```python
from build123d import *

# Parameters (mm, degrees)
F0_W          = 1463
F0_H          = 50
F1_DEPTH      = 15
F1_DEPTH_BACK = 15
F3_DEPTH      = 50
F5_DEPTH      = 50


with BuildPart() as f1:
    # F0 (on Right) → F1 (new body, two sides)
    with BuildSketch(Plane.YZ) as f1_sk:
        Rectangle(F0_W, F0_H)
    extrude(amount=F1_DEPTH)
    extrude(f1_sk.sketch, amount=-F1_DEPTH_BACK)

    # F2 (on face) → F3 (join)
    with BuildSketch(Plane(origin=(0, 0, -25), x_dir=(1, 0, 0), z_dir=(0, 0, -1))):
        with BuildLine():
            ThreePointArc((0, 729.5), (-4.949747, 717.550253), (7, 722.5))
            ThreePointArc((7, 722.5), (4.949747, 727.449747), (0, 729.5))
        make_face()
    extrude(amount=F3_DEPTH)

    # F4 (on face) → F5 (join)
    with BuildSketch(Plane(origin=(0, 0, -25), x_dir=(1, 0, 0), z_dir=(0, 0, -1))):
        with BuildLine():
            ThreePointArc((0, -729.5), (4.949747, -727.449747), (7, -722.5))
            ThreePointArc((7, -722.5), (-4.949747, -717.550253), (0, -729.5))
        make_face()
    extrude(amount=F5_DEPTH)


solid = f1.part
```
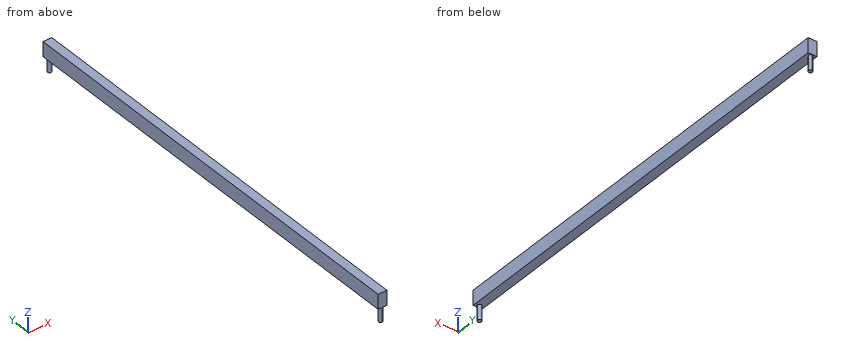
Geometry check sheet. Reference: the model listing, model coordinates, mm. Coordinates: 2 decimals unless noted, no trailing zeros. Write each loop counter-clockwise with the first axis right and the second up, starting at its lowest first coordinate (ties: lowest second). Pieces come first, ordered by that corner, then holes. Notation, with made-up numbers: M 50.25,66 L 109.25,66 A14 ccw 109.25,84 Z; hole C 48.25,7.5 d9. An arc over 180 degrees is marked long. One line per item, written item: value. Start each with the question number.
(1) Sectioned sample at B-B, the plane y = -636.5. Enter the section's corners in (x, z), and give its area (3 significant figures).
(2) Scan lines: line 1 along Y through (x, z) = (1.75, -67); line 2 along Z through (x, y) = (-8, -433.5); line 3 along Y through (x, z) = (4.25, -56). Record each from-to range of solid material in increasing order. Write a range as [from, to].
(3) Depth check by flat-ended pin: pin 1 (5 mm diameter, centred on x = -7.5, z = -56.5, fed in from +Y); pin 2 (2 mm diameter, centred on x = 6, y = -391.5, fed in from -Z). Enter the tip coordinate at first touch or a pass-through.
(4) Sectioned sample at A-A, the plane z = -59.5. Enter the section's corners in (x, y).
Filled sheet:
1. outline: M -15,-25 L 15,-25 L 15,25 L -15,25 Z
1. area: 1,500 mm²
2. line 1: [-729.28, -715.72], [715.72, 729.28]
2. line 2: [-25, 25]
2. line 3: [-728.06, -716.94], [716.94, 728.06]
3. pin 1: y = 727.4
3. pin 2: z = -25
4. outline: M 0,-729.5 A7 ccw 7,-722.5 A7 ccw long Z; M 0,729.5 A7 ccw long 7,722.5 A7 ccw Z
